Could you check a few things on this model? Use its own coordinates, in mm. A direction names the side the tool comes from. Coordinates: 2 decimals unless noted, no trailing zeros. Order: outer loops, then holes, each group sorted by start corner. A loop starts at its lowest first (then second) coordinate and runs counter-clockwise, first axis right, second up. Notation, with made-up numbers: M 67,69 L 101,69 A22 ccw 101,88 Z; hole C -32.5,51 d8. An arc over 180 degrees is marked long. Put each result on its own line as item: value. Start each with the question number.
```python
from build123d import *

# Parameters (mm, degrees)
F0_R     = 1.5875
F1_DEPTH = 3.175
F3_DEPTH = 3.176


with BuildPart() as f1:
    # F0 (on Front) → F1 (new body)
    with BuildSketch(Plane.XZ):
        with BuildLine():
            Line((-22.31495, 34.72274), (-23.197748, 30.22374))
            ThreePointArc((-23.197748, 30.22374), (-24.950194, 28.794059), (-26.614722, 27.262915))
            Line((-26.614722, 27.262915), (-31.193564, 27.029377))
            Line((-31.193564, 27.029377), (-30.773088, 22.463906))
            ThreePointArc((-30.773088, 22.463906), (-32.05176, 20.598415), (-33.21749, 18.660342))
            Line((-33.21749, 18.660342), (-37.545061, 17.146255))
            Line((-37.545061, 17.146255), (-35.855375, 12.884179))
            ThreePointArc((-35.855375, 12.884179), (-36.556682, 10.73401), (-37.129174, 8.546019))
            Line((-37.129174, 8.546019), (-40.85488, 5.874045))
            Line((-40.85488, 5.874045), (-38.032873, 2.260652))
            ThreePointArc((-38.032873, 2.260652), (-38.1, 0), (-38.032873, -2.260652))
            Line((-38.032873, -2.260652), (-40.85488, -5.874045))
            Line((-40.85488, -5.874045), (-37.129174, -8.546019))
            ThreePointArc((-37.129174, -8.546019), (-36.556682, -10.73401), (-35.855375, -12.884179))
            Line((-35.855375, -12.884179), (-37.545061, -17.146255))
            Line((-37.545061, -17.146255), (-33.21749, -18.660342))
            ThreePointArc((-33.21749, -18.660342), (-32.05176, -20.598415), (-30.773088, -22.463906))
            Line((-30.773088, -22.463906), (-31.193564, -27.029377))
            Line((-31.193564, -27.029377), (-26.614722, -27.262915))
            ThreePointArc((-26.614722, -27.262915), (-24.950194, -28.794059), (-23.197748, -30.22374))
            Line((-23.197748, -30.22374), (-22.31495, -34.72274))
            Line((-22.31495, -34.72274), (-17.855788, -33.656809))
            ThreePointArc((-17.855788, -33.656809), (-15.827312, -34.656979), (-13.743065, -35.535027))
            Line((-13.743065, -35.535027), (-11.628511, -39.603072))
            Line((-11.628511, -39.603072), (-7.650284, -37.324029))
            ThreePointArc((-7.650284, -37.324029), (-5.422195, -37.712197), (-3.175, -37.967478))
            Line((-3.175, -37.967478), (0, -41.275))
            Line((0, -41.275), (3.175, -37.967478))
            ThreePointArc((3.175, -37.967478), (5.422195, -37.712197), (7.650284, -37.324029))
            Line((7.650284, -37.324029), (11.628511, -39.603072))
            Line((11.628511, -39.603072), (13.743065, -35.535027))
            ThreePointArc((13.743065, -35.535027), (15.827312, -34.656979), (17.855788, -33.656809))
            Line((17.855788, -33.656809), (22.31495, -34.72274))
            Line((22.31495, -34.72274), (23.197748, -30.22374))
            ThreePointArc((23.197748, -30.22374), (24.950194, -28.794059), (26.614722, -27.262915))
            Line((26.614722, -27.262915), (31.193564, -27.029377))
            Line((31.193564, -27.029377), (30.773088, -22.463906))
            ThreePointArc((30.773088, -22.463906), (32.05176, -20.598415), (33.21749, -18.660342))
            Line((33.21749, -18.660342), (37.545061, -17.146255))
            Line((37.545061, -17.146255), (35.855375, -12.884179))
            ThreePointArc((35.855375, -12.884179), (36.556682, -10.73401), (37.129174, -8.546019))
            Line((37.129174, -8.546019), (40.85488, -5.874045))
            Line((40.85488, -5.874045), (38.032873, -2.260652))
            ThreePointArc((38.032873, -2.260652), (38.1, 0), (38.032873, 2.260652))
            Line((38.032873, 2.260652), (40.85488, 5.874045))
            Line((40.85488, 5.874045), (37.129174, 8.546019))
            ThreePointArc((37.129174, 8.546019), (36.556682, 10.73401), (35.855375, 12.884179))
            Line((35.855375, 12.884179), (37.545061, 17.146255))
            Line((37.545061, 17.146255), (33.21749, 18.660342))
            ThreePointArc((33.21749, 18.660342), (32.05176, 20.598415), (30.773088, 22.463906))
            Line((30.773088, 22.463906), (31.193564, 27.029377))
            Line((31.193564, 27.029377), (26.614722, 27.262915))
            ThreePointArc((26.614722, 27.262915), (24.950194, 28.794059), (23.197748, 30.22374))
            Line((23.197748, 30.22374), (22.31495, 34.72274))
            Line((22.31495, 34.72274), (17.855788, 33.656809))
            ThreePointArc((17.855788, 33.656809), (15.827312, 34.656979), (13.743065, 35.535027))
            Line((13.743065, 35.535027), (11.628511, 39.603072))
            Line((11.628511, 39.603072), (7.650284, 37.324029))
            ThreePointArc((7.650284, 37.324029), (5.422195, 37.712197), (3.175, 37.967478))
            Line((3.175, 37.967478), (0, 41.275))
            Line((0, 41.275), (-3.175, 37.967478))
            ThreePointArc((-3.175, 37.967478), (-5.422195, 37.712197), (-7.650284, 37.324029))
            Line((-7.650284, 37.324029), (-11.628511, 39.603072))
            Line((-11.628511, 39.603072), (-13.743065, 35.535027))
            ThreePointArc((-13.743065, 35.535027), (-15.827312, 34.656979), (-17.855788, 33.656809))
            Line((-17.855788, 33.656809), (-22.31495, 34.72274))
        make_face()
        with Locations((-21.997045, -12.7)):
            Circle(F0_R, mode=Mode.SUBTRACT)
        with Locations((0, -25.4)):
            Circle(F0_R, mode=Mode.SUBTRACT)
        with Locations((21.997045, -12.7)):
            Circle(F0_R, mode=Mode.SUBTRACT)
        with Locations((-21.997045, 12.7)):
            Circle(F0_R, mode=Mode.SUBTRACT)
        with Locations((21.997045, 12.7)):
            Circle(F0_R, mode=Mode.SUBTRACT)
        with Locations((0, 25.4)):
            Circle(F0_R, mode=Mode.SUBTRACT)
    extrude(amount=F1_DEPTH)

    # F2 (on face) → F3 (cut, through all)
    with BuildSketch(Plane.XZ.offset(3.175)):
        Polygon((3.666174, 6.35), (-3.666174, 6.35), (-7.332348, 0), (-3.666174, -6.35), (3.666174, -6.35), (7.332348, 0), align=None)
    extrude(amount=-F3_DEPTH, mode=Mode.SUBTRACT)


solid = f1.part
```
Item 1: If we section it at C-C on z = 4: Write out the boundary of the cut face in (x, y) (3 decimals), then the cut area to 3 significant figures.
Item 2: For pin 1 Ø1.5 at (y, z) = (-2.5, -27) entering from -X; pin 2 Ø1.6 at (x, y) = (-1.5, -1.5) entering from -Z; pin 3 Ø1.9 at (x, z) = (-22, 12.7) entering from -Y; pin 4 Ø1.5 at (y, z) = (-2, -11.5) entering from +X, each with a flat end and sliding along its axis, tell me the tip position at first contact or that it passes through.
Item 3: If we mould it in two halves opening along X, with no side actions, what happens to faces 1 (the flat face through (-12.67, -1.57, 37.6)), 2 (the flat face through (1.61, -1.57, 39.6)), 3 (the cylindrical face through (24.93, -1.57, -28.81))? For each: released by +X, released by -X, zero draft, split by the parting line, or undercut.
Item 4: If we section it at B-B on y = -2.6: State how many separate pieces and enclosed holes the cut face has, then the cut area to 3 significant figures.
Item 5: If we section it at A-A on z = 25.4: Write out the boundary of the cut face in (x, y) (1 decimal), then the cut area to 3 significant figures.
Item 6: If we section it at D-D on z = -16: Write out the boundary of the cut face in (x, y) (3 decimals).
Item 7: I need wall thicknesses on probe 1 along X at (y, z) = (-2.25, -12); probe 2 along X at (y, z) = (-0.65, -5.5); probe 3 along Z at (x, y) = (1, -0.45). Which ranges of each line are inside material? Lowest first, please.
Item 8: For faces 4 (the flat face through (5.474, -1.61, -3.219)), 5 (the flat face through (-30.986, -1.565, 24.779)), 6 (the flat face through (1.57, -1.57, -39.64)), 7 (the cylindrical face through (-15.8, -1.57, 34.67)), which set-ups out of +Z, -Z, +X, -X, +Y, -Y let a thin tool reach every point of the face, with its end or its side?
Geometry check:
1. outline: M -39.391,-3.175 L -5.023,-3.175 L -5.023,0 L -39.391,0 Z; M 5.023,-3.175 L 39.391,-3.175 L 39.391,0 L 5.023,0 Z
1. area: 218 mm²
2. pin 1: stops at x = -31.19
2. pin 2: stops at z = -40.55
2. pin 3: passes through
2. pin 4: stops at x = 36.55
3. face 1: released by -X
3. face 2: undercut
3. face 3: released by +X
4. separate pieces: 1
4. enclosed holes: 7
4. area: 4,590 mm²
5. outline: M -31,-3.2 L -1.6,-3.2 L -1.6,0 L -31,0 Z; M 1.6,-3.2 L 31,-3.2 L 31,0 L 1.6,0 Z
5. area: 187 mm²
6. outline: M -37.091,-3.175 L 37.091,-3.175 L 37.091,0 L -37.091,0 Z
7. probe 1: x = -36.16 to -23.42, -20.57 to 20.57, 23.42 to 36.16
7. probe 2: x = -40.56 to -4.16, 4.16 to 40.56
7. probe 3: z = -40.23 to -26.63, -24.17 to -6.35, 6.35 to 24.17, 26.63 to 40.23
8. face 4: +Y, -Y
8. face 5: -X, +Y, -Y
8. face 6: -Z, +Y, -Y
8. face 7: +Z, +Y, -Y
